Read the model definition and answer for the solid it produces. Units are mm, in the model's axes. Face numbers are marked on the shaded views. A direction names the side the tool comes from. Give positions to 0.01 mm unless a question says otherwise; leave off trailing zeros. Loops run counter-clockwise (first coordinate to the right, second up) from the corner with the lowest first, then second, coordinate; pieces in that order, holes last. Notation, with made-up numbers: (56.5, 0) - (84.5, 0) arc R22 ccw to (84.5, 37) - close; hole circle Ø3 at (-35.5, 6). An arc over 180 degrees is marked (long way). Write each question's results on one line, items separated by ' | '. Start each with the question number.
Q1. The part is cut by section D-D, the plane z = 11.75. Write down the section's boundary in (x, y).
Q2. For the marked faces 4, 5 and 6, determine the directions among +Z, -Z, +X, -X, +Y, -Y from which every point of the face is accessible in a straight line to the end or side of a thin tool.
Q3. The part is cut by section B-B, the plane x = 2.5. Write down the section's boundary in (y, z).
Q4. Determine the mould class of the marked faces 1, 2 and 3 for opening direction X: +X half, -X half, draft (parallel to the pull), parting line (faces both ways), or undercut.
Q5. Given pin 1 (7.5 mm diameter, centred on y = -2, z = 6, fed in from -X); pin 2 (6 mm diameter, centred on x = -11.5, z = 9, fed in from +Y); pin 3 (2.5 mm diameter, centred on x = -10.5, z = 6.5, fed in from +Y), each flat-ended and moving along its own axis, determine where each tip first touches the part or whether it passes through.
Q6. The part is cut by section C-C, the plane x = -11.25. Write down the section's boundary in (y, z).
Q7. The part is cut by section A-A, the plane y = -1.15. Write down the section's boundary in (x, z).
Q8. Find the intervals of material crossed by line 1 (X direction, y = -1.15, z = 8); line 2 (Z direction, x = 6.25, y = 6); line 3 (Z direction, x = 2.75, y = 6), in increasing order. Write a range as from..to.
```python
from build123d import *

# Parameters (mm, degrees)
F0_R      = 4.15
F1_DEPTH  = 15
F2_W      = 1
F2_H      = 15
F3_DEPTH  = 10
F6_D      = 3.5
F7_R      = 1.75
F8_DEPTH  = 25
F4_R      = 1.75
F9_DEPTH  = 22.501
F10_R     = 1.75
F11_DEPTH = 2.5
F4_R_2    = 2.7
F12_DEPTH = 2.6
F7_R_2    = 2.7
F13_DEPTH = 3
F5_R      = 2.7
F5_R_2    = 1.75
F14_DEPTH = 3


with BuildPart() as f1:
    # F0 (on Top) → F1 (new body)
    with BuildSketch(Plane.XY):
        Polygon((7.5, 10), (-7.5, 10), (-7.5, -10), (-15, -10), (-15, -16), (15, -16), (15, -10), (7.5, -10), align=None)
        with Locations((0, -1.15)):
            Circle(F0_R, mode=Mode.SUBTRACT)
    extrude(amount=F1_DEPTH)

    # F2 (on face) → F3 (cut)
    with BuildSketch(Plane(origin=(0, 10, 0), x_dir=(-1, 0, 0), z_dir=(0, 1, 0))):
        with Locations((0, 7.5)):
            Rectangle(F2_W, F2_H)
    extrude(amount=-F3_DEPTH, mode=Mode.SUBTRACT)

    # F6 (through all)
    with Locations(Plane(origin=(0, -10, 0), x_dir=(-1, 0, 0), z_dir=(0, 1, 0))):
        with Locations((-11.25, 7.5)):
            Hole(F6_D / 2)

    # F7 (on face) → F8 (cut)
    with BuildSketch(Plane(origin=(0, -10, 0), x_dir=(-1, 0, 0), z_dir=(0, 1, 0))):
        with Locations((11.25, 7.5)):
            Circle(F7_R)
    extrude(amount=-F8_DEPTH, mode=Mode.SUBTRACT)

    # F4 (on face) → F9 (cut, through all)
    with BuildSketch(Plane.YZ.offset(7.5)):
        with Locations((6, 7.5)):
            Circle(F4_R)
    extrude(amount=-F9_DEPTH, mode=Mode.SUBTRACT)

    # F10 (on face) → F11 (cut)
    with BuildSketch(Plane(origin=(-7.5, 0, 0), x_dir=(0, -1, 0), z_dir=(-1, 0, 0))):
        Polygon((-7.151114, 10.521303), (-9.192082, 8.013758), (-8.040968, 4.992455), (-4.848886, 4.478697), (-2.807918, 6.986242), (-3.959032, 10.007545), align=None)
        with Locations((-6, 7.5)):
            Circle(F10_R, mode=Mode.SUBTRACT)
    extrude(amount=-F11_DEPTH, mode=Mode.SUBTRACT)

    # F4 (on face) → F12 (cut)
    with BuildSketch(Plane.YZ.offset(7.5)):
        with Locations((6, 7.5)):
            Circle(F4_R_2)
        with Locations((6, 7.5)):
            Circle(F4_R, mode=Mode.SUBTRACT)
    extrude(amount=-F12_DEPTH, mode=Mode.SUBTRACT)

    # F7 (on face) → F13 (cut)
    with BuildSketch(Plane(origin=(0, -10, 0), x_dir=(-1, 0, 0), z_dir=(0, 1, 0))):
        with Locations((11.25, 7.5)):
            Circle(F7_R_2)
        with Locations((11.25, 7.5)):
            Circle(F7_R, mode=Mode.SUBTRACT)
    extrude(amount=-F13_DEPTH, mode=Mode.SUBTRACT)

    # F5 (on face) → F14 (cut)
    with BuildSketch(Plane(origin=(0, -10, 0), x_dir=(-1, 0, 0), z_dir=(0, 1, 0))):
        with Locations((-11.25, 7.5)):
            Circle(F5_R)
        with Locations((-11.25, 7.5)):
            Circle(F5_R_2, mode=Mode.SUBTRACT)
    extrude(amount=-F14_DEPTH, mode=Mode.SUBTRACT)


solid = f1.part
```
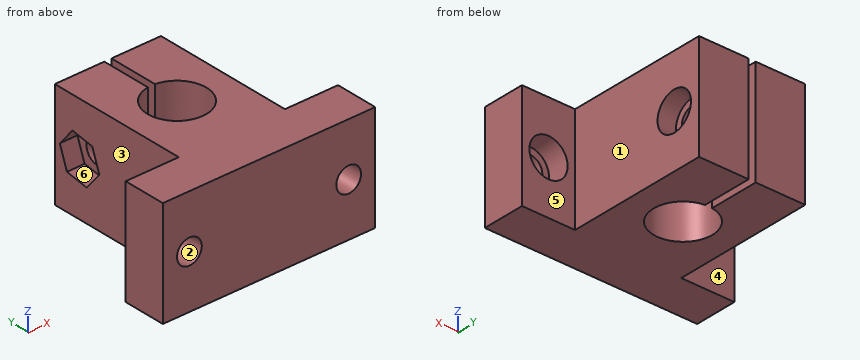
Check sheet entries:
1) outline: (-15, -16) - (15, -16) - (15, -10) - (7.5, -10) - (7.5, 10) - (0.5, 10) - (0.5, 2.97) arc R4.15 cw (long way) to (-0.5, 2.97) - (-0.5, 10) - (-7.5, 10) - (-7.5, -10) - (-15, -10) - close
2) face 4: +Z, -Z, -X, +Y | face 5: +Z, -Z, +X, +Y | face 6: -X
3) outline: (-16, 0) - (-4.46, 0) - (-4.46, 15) - (-16, 15) - close; (2.16, 0) - (10, 0) - (10, 15) - (2.16, 15) - close; hole circle Ø3.5 at (6, 7.5)
4) face 1: +X half | face 2: undercut | face 3: -X half
5) pin 1: stops at x = -7.5 | pin 2: stops at y = -10 | pin 3: stops at y = -13
6) outline: (-16, 0) - (-10, 0) - (-10, 4.8) - (-13, 4.8) - (-13, 5.75) - (-16, 5.75) - close; (-16, 9.25) - (-13, 9.25) - (-13, 10.2) - (-10, 10.2) - (-10, 15) - (-16, 15) - close
7) outline: (-7.5, 0) - (-4.15, 0) - (-4.15, 15) - (-7.5, 15) - close; (4.15, 0) - (7.5, 0) - (7.5, 15) - (4.15, 15) - close
8) line 1: x = -7.5..-4.15, 4.15..7.5 | line 2: z = 0..4.8, 10.2..15 | line 3: z = 0..5.75, 9.25..15
